Part model, mm, in its own coordinate system. A direction names the side the tool comes from. Give positions to 0.01 mm unless a question says otherwise; leave off trailing zeros. Order: outer loops, then holes, each group sorted by start corner. A loop starts at its lowest first (then second) coordinate and runs counter-clockwise, first axis right, second up.
1. Slice it at B-B on y = -211.5. List the corners of the cut face in (x, z), and give its area (3 significant figures).
2. Probe line 1 (Y direction, x = -76.5, z = 10.25); line 2 (X direction, y = -171.5, z = 0.5); line 3 (Z direction, x = -205.5, y = 169). List the from-to ranges inside material, lowest first.
3. Drop flat-ended pins along their axis: pin 1 Ø8 at (x, y) = (218.5, 241.5) entering from +Z; pin 2 Ø1 at (x, z) = (-71, 10.5) entering from -Y; pin 3 Ø6 at (x, z) = (-149, 3.5) entering from +Y; pin 4 Ø5 at (x, y) = (-132.5, -88) entering from +Z. Give the stop position or say it passes through.
4. Mould opens along X. For faces 4 (the flat face through (222, 238, 9.7)), 5 (the flat face through (-230, -3, 2)), 6 (the cylindrical face through (-2.996, 248.834, 0.183)), 7 (the flat face through (-3, -9, 9.7)) say: +X half, -X half, draft (parallel to the pull), parting line (faces both ways), or undercut.
5. Slice it at D-D on y = 242. List the corners of the cut face in (x, z), and give its area (3 significant figures).
6. Slice it at A-A on x = 165.5. List the corners of the cut face in (y, z).
7. Which spindle directions (+Z, -Z, +X, -X, +Y, -Y) get a long thin tool onto all of the face, cutting with end or side? Do faces 1 (the flat face through (-3, -169, 9.7)), 2 (the flat face through (-3, -169, 10.9)), 3 (the flat face through (-222, 238, 9.7)). Say none if no direction does.
8. Slice it at C-C on z = 1.7. List the corners of the cut face in (x, y).
from build123d import *

# Parameters (mm, degrees)
SKETCH1_W             = 16
SKETCH1_H             = 16
BOSS_EXTRUDE1_DEPTH   = 250
BOSS_EXTRUDE1_2_DEPTH = 250
SKETCH2_W             = 460
SKETCH2_H             = 150
BOSS_EXTRUDE2_DEPTH   = 1.2
SKETCH3_R             = 7
BOSS_EXTRUDE3_DEPTH   = 428


with BuildPart() as part:
    # Sketch1 → Boss-Extrude1 (new, symmetric)
    with BuildSketch(Plane(origin=(0, 0, 0), x_dir=(1, 0, 0), z_dir=(0, 1, 0))):
        with Locations((-222, -1.7)):
            Rectangle(SKETCH1_W, SKETCH1_H)
    extrude(amount=BOSS_EXTRUDE1_DEPTH, both=True)



with BuildPart() as body_2:
    # Sketch1 → Boss-Extrude1 2 (new, symmetric)
    with BuildSketch(Plane(origin=(0, 0, 0), x_dir=(1, 0, 0), z_dir=(0, 1, 0))):
        with Locations((222, -1.7)):
            Rectangle(SKETCH1_W, SKETCH1_H)
    extrude(amount=BOSS_EXTRUDE1_2_DEPTH, both=True)


with BuildPart() as part_1:
    add(part.part)

    add(body_2.part)  # Boss-Extrude2 merges body 2
    # Sketch2 → Boss-Extrude2 (add)
    with BuildSketch(Plane.XY.offset(9.7)):
        with Locations((0, 150)):
            Rectangle(SKETCH2_W, SKETCH2_H)
        with Locations((0, -10)):
            Rectangle(SKETCH2_W, SKETCH2_H)
        with Locations((0, -170)):
            Rectangle(SKETCH2_W, SKETCH2_H)
    extrude(amount=BOSS_EXTRUDE2_DEPTH)

    # Sketch3 → Boss-Extrude3 (add)
    with BuildSketch(Plane(origin=(-214, 0, 0), x_dir=(0, 0, -1), z_dir=(1, 0, 0))):
        with Locations(Location((-1.7, 242, 0), (0, 0, 180))):
            Circle(SKETCH3_R)
    extrude(amount=BOSS_EXTRUDE3_DEPTH)


solid = part_1.part
Data:
1. outline: (-230, -6.3) - (-214, -6.3) - (-214, 9.7) - (214, 9.7) - (214, -6.3) - (230, -6.3) - (230, 10.9) - (-230, 10.9) - close
1. area: 1,060 mm2
2. line 1: y = -245 to -95, -85 to 65, 75 to 225
2. line 2: x = -230 to -214, 214 to 230
2. line 3: z = 9.7 to 10.9
3. pin 1: stops at z = 9.7
3. pin 2: stops at y = -245
3. pin 3: stops at y = 249
3. pin 4: passes through
4. face 4: draft
4. face 5: -X half
4. face 6: undercut
4. face 7: undercut
5. outline: (-230, -6.3) - (-214, -6.3) - (-214, -5.3) - (214, -5.3) - (214, -6.3) - (230, -6.3) - (230, 9.7) - (214, 9.7) - (214, 8.7) - (-214, 8.7) - (-214, 9.7) - (-230, 9.7) - close
5. area: 6,500 mm2
6. outline: (-245, 9.7) - (-95, 9.7) - (-95, 10.9) - (-245, 10.9) - close; (-85, 9.7) - (65, 9.7) - (65, 10.9) - (-85, 10.9) - close; (75, 9.7) - (225, 9.7) - (225, 10.9) - (75, 10.9) - close; circle Ø14 at (242, 1.7)
7. face 1: -Z, +Y, -Y
7. face 2: +Z, +X, -X, +Y, -Y
7. face 3: +Z, +X, -X, +Y
8. outline: (-230, -250) - (-214, -250) - (-214, 235) - (214, 235) - (214, -250) - (230, -250) - (230, 250) - (214, 250) - (214, 249) - (-214, 249) - (-214, 250) - (-230, 250) - close
